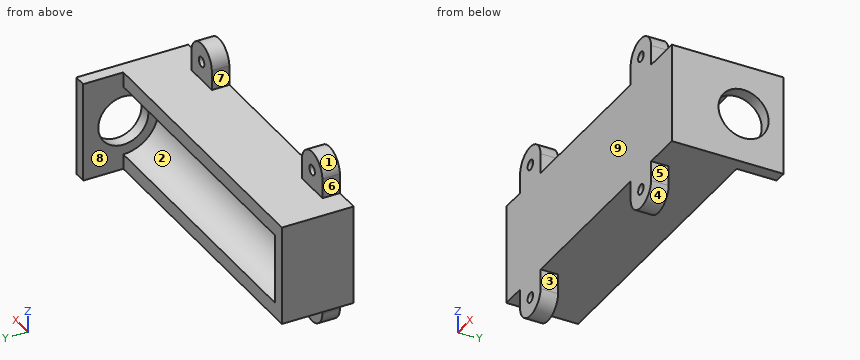
```python
from build123d import *

# Parameters (mm, degrees)
BOSS_EXTRUDE1_DEPTH     = 55.3
SKETCH3_W               = 40
SKETCH3_H               = 19
BOSS_EXTRUDE2_DEPTH     = 5
SKETCH5_R               = 10
CUT_EXTRUDE1_DEPTH      = 10
SKETCH6_W               = 15
SKETCH6_H               = 15
SKETCH6_R               = 2
BOSS_EXTRUDE3_DEPTH     = 5
BOSS_EXTRUDE3_2_DEPTH   = 5
BOSS_EXTRUDE3_3_DEPTH   = 5
BOSS_EXTRUDE3_4_DEPTH   = 5
FILLET5_R               = 7
FILLET2_R               = 7
FILLET3_R               = 7
FILLET4_R               = 7
BOSS_EXTRU_1_START      = 110.6
BOSS_EXTRU_1_DEPTH      = 110.6
ESQUISSE11_W            = 40
ESQUISSE11_H            = 9.66
BOSS_EXTRU_5_DEPTH      = 120.6
ESQUISSE12_R            = 2.003722313
ESQUISSE12_R_2          = 2
BOSS_EXTRU_6_DEPTH      = 7
ESQUISSE13_W            = 97.971196864
ESQUISSE13_H            = 26.942074747
ENL_V_MAT_EXTRU_2_DEPTH = 20
ESQUISSE16_R            = 2
ENL_V_MAT_EXTRU_3_DEPTH = 20
BOSS_EXTRU_7_DEPTH      = 5


with BuildPart() as part:
    # Sketch1 → Boss-Extrude1 (new, symmetric)
    with BuildSketch(Plane(origin=(0, 0, 0), x_dir=(0, 0, -1), z_dir=(1, 0, 0))):
        with BuildLine():
            ThreePointArc((-15, 0), (0, -15), (15, 0))
            Line((15, 0), (20, 0))
            Line((20, 0), (20, -19))
            Line((20, -19), (-20, -19))
            Line((-20, -19), (-20, 0))
            Line((-20, 0), (-15, 0))
        make_face()
    extrude(amount=BOSS_EXTRUDE1_DEPTH, both=True)

    # Sketch3 → Boss-Extrude2 (add)
    with BuildSketch(Plane(origin=(55.3, 0, 0), x_dir=(0, 0, -1), z_dir=(1, 0, 0))):
        with Locations((0, -9.5)):
            Rectangle(SKETCH3_W, SKETCH3_H)
    boss_extrude2 = extrude(amount=BOSS_EXTRUDE2_DEPTH)

    # Mirror1: Boss-Extrude2 across plane
    add(boss_extrude2.mirror(Plane(origin=(0, 0, 0), x_dir=(0, 0, 1), z_dir=(1, 0, 0))))

    # Sketch5 → Cut-Extrude1 (cut)
    with BuildSketch(Plane(origin=(60.3, 0, 0), x_dir=(0, 0, -1), z_dir=(1, 0, 0))):
        Circle(SKETCH5_R)
    extrude(amount=-CUT_EXTRUDE1_DEPTH, mode=Mode.SUBTRACT)

    # Esquisse3 → Boss.-Extru.1 (add)
    with BuildSketch(Plane(origin=(-55.3, 0, 0), x_dir=(0, 0, -1), z_dir=(1, 0, 0)).offset(BOSS_EXTRU_1_START)):
        with BuildLine():
            Line((-15, 0), (-14, 0))
            ThreePointArc((-14, 0), (0, -14), (14, 0))
            Line((14, 0), (15, 0))
            ThreePointArc((15, 0), (0, -15), (-15, 0))
        make_face()
    extrude(amount=-BOSS_EXTRU_1_DEPTH)



with BuildPart() as body_2:
    # Sketch6 → Boss-Extrude3 (new body)
    with BuildSketch(Plane.XZ.offset(19)):
        with Locations((37.8, 27.5)):
            Rectangle(SKETCH6_W, SKETCH6_H)
        with Locations(Location((37.8, 27.5, 0), (0, 0, 270))):
            Circle(SKETCH6_R, mode=Mode.SUBTRACT)
    extrude(amount=-BOSS_EXTRUDE3_DEPTH)

    # Fillet5
    fillet5_edges = [body_2.edges().sort_by_distance(p)[0] for p in [
        (30.3, -16.5, 35),
        (45.3, -16.5, 35),
    ]]
    fillet(fillet5_edges, radius=FILLET5_R)


with BuildPart() as body_3:
    # Sketch6 → Boss-Extrude3 2 (new body)
    with BuildSketch(Plane.XZ.offset(19)):
        with Locations((-42.8, 27.5)):
            Rectangle(SKETCH6_W, SKETCH6_H)
        with Locations(Location((-42.8, 27.5, 0), (0, 0, 270))):
            Circle(SKETCH6_R, mode=Mode.SUBTRACT)
    extrude(amount=-BOSS_EXTRUDE3_2_DEPTH)

    # Fillet2
    fillet2_edges = [body_3.edges().sort_by_distance(p)[0] for p in [
        (-35.3, -16.5, 35),
        (-50.3, -16.5, 35),
    ]]
    fillet(fillet2_edges, radius=FILLET2_R)


with BuildPart() as body_4:
    # Sketch6 → Boss-Extrude3 3 (new body)
    with BuildSketch(Plane.XZ.offset(19)):
        with Locations((37.8, -27.5)):
            Rectangle(SKETCH6_W, SKETCH6_H)
        with Locations(Location((37.8, -27.5, 0), (0, 0, 90))):
            Circle(SKETCH6_R, mode=Mode.SUBTRACT)
    extrude(amount=-BOSS_EXTRUDE3_3_DEPTH)

    # Fillet4
    fillet4_edges = [body_4.edges().sort_by_distance(p)[0] for p in [
        (30.3, -16.5, -35),
        (45.3, -16.5, -35),
    ]]
    fillet(fillet4_edges, radius=FILLET4_R)


with BuildPart() as body_5:
    # Sketch6 → Boss-Extrude3 4 (new body)
    with BuildSketch(Plane.XZ.offset(19)):
        with Locations((-42.8, -27.5)):
            Rectangle(SKETCH6_W, SKETCH6_H)
        with Locations(Location((-42.8, -27.5, 0), (0, 0, 90))):
            Circle(SKETCH6_R, mode=Mode.SUBTRACT)
    extrude(amount=-BOSS_EXTRUDE3_4_DEPTH)

    # Fillet3
    fillet3_edges = [body_5.edges().sort_by_distance(p)[0] for p in [
        (-50.3, -16.5, -35),
        (-35.3, -16.5, -35),
    ]]
    fillet(fillet3_edges, radius=FILLET3_R)


with BuildPart() as part_1:
    add(part.part)

    add(body_2.part)  # Boss.-Extru.5 merges body 2

    add(body_3.part)  # Boss.-Extru.5 merges body 3

    add(body_4.part)  # Boss.-Extru.5 merges body 4

    add(body_5.part)  # Boss.-Extru.5 merges body 5
    # Esquisse11 → Boss.-Extru.5 (add)
    with BuildSketch(Plane.ZY.offset(60.3)):
        with Locations((0, -23.83)):
            Rectangle(ESQUISSE11_W, ESQUISSE11_H)
    extrude(amount=-BOSS_EXTRU_5_DEPTH)

    # Esquisse12 → Boss.-Extru.6 (add)
    # profile 1 of 4: a face of its own
    with BuildSketch(Plane.XZ.offset(28.66)):
        with BuildLine():
            Line((-50.3, 28), (-50.3, 20))
            Line((-50.3, 20), (-35.3, 20))
            Line((-35.3, 20), (-35.3, 28))
            ThreePointArc((-35.3, 28), (-42.8, 35.016648189), (-50.3, 28))
        make_face()
        with Locations(Location((-42.8, 27.5, 0), (0, 0, 270))):
            Circle(ESQUISSE12_R, mode=Mode.SUBTRACT)
    # profile 2 of 4: a face of its own
    with BuildSketch(Plane.XZ.offset(28.66)):
        with BuildLine():
            Line((-35.3, -20), (-50.3, -20))
            Line((-50.3, -20), (-50.3, -28))
            ThreePointArc((-50.3, -28), (-42.8, -35.016648189), (-35.3, -28))
            Line((-35.3, -28), (-35.3, -20))
        make_face()
    # profile 3 of 4: a face of its own
    with BuildSketch(Plane.XZ.offset(28.66)):
        with BuildLine():
            Line((45.3, -20), (30.3, -20))
            Line((30.3, -20), (30.3, -28))
            ThreePointArc((30.3, -28), (37.8, -35.016648189), (45.3, -28))
            Line((45.3, -28), (45.3, -20))
        make_face()
        with Locations(Location((37.8, -27.5, 0), (0, 0, 90))):
            Circle(ESQUISSE12_R_2, mode=Mode.SUBTRACT)
    # profile 4 of 4: a face of its own
    with BuildSketch(Plane.XZ.offset(28.66)):
        with BuildLine():
            Line((30.3, 28), (30.3, 20))
            Line((30.3, 20), (45.3, 20))
            Line((45.3, 20), (45.3, 28))
            ThreePointArc((45.3, 28), (37.8, 35.016648189), (30.3, 28))
        make_face()
        with Locations(Location((37.8, 27.5, 0), (0, 0, 270))):
            Circle(ESQUISSE12_R_2, mode=Mode.SUBTRACT)
    extrude(amount=-BOSS_EXTRU_6_DEPTH)

    # Esquisse13 → Enlèv. mat.-Extru.2 (cut)
    with BuildSketch(Plane(origin=(0, 0, 0), x_dir=(1, 0, 0), z_dir=(0, 1, 0))):
        Polygon((-50.3, -20), (-50.3, -48.328087832), (45.678803054, -48.328087832), (45.3, -20), align=None)
        with Locations((-1.314401568, 33.471037373)):
            Rectangle(ESQUISSE13_W, ESQUISSE13_H)
    extrude(amount=-ENL_V_MAT_EXTRU_2_DEPTH, mode=Mode.SUBTRACT)

    # Esquisse16 → Enlèv. mat.-Extru.3 (cut)
    with BuildSketch(Plane.XZ.offset(28.66)):
        with Locations(Location((-42.8, -27.5, 0), (0, 0, 270))):
            Circle(ESQUISSE16_R)
    extrude(amount=-ENL_V_MAT_EXTRU_3_DEPTH, mode=Mode.SUBTRACT)

    # Esquisse18 → Boss.-Extru.7 (add)
    with BuildSketch(Plane(origin=(60.3, 0, 0), x_dir=(0, 0, -1), z_dir=(1, 0, 0))):
        with BuildLine():
            Line((-20, 0), (-20, 16))
            Line((-20, 16), (20, 16))
            Line((20, 16), (20, 0))
            Line((20, 0), (10, 0))
            ThreePointArc((10, 0), (0, 10), (-10, 0))
            Line((-10, 0), (-20, 0))
        make_face()
    extrude(amount=-BOSS_EXTRU_7_DEPTH)


solid = part_1.part
```
CAD build for the part. Positions are in the model's coordinates, mm. Face numbers are marked on the shaded views. A direction names the side the tool comes from. Round coordinates to 2 decimals unless told otherwise and drop trailing zeros. Loops run counter-clockwise (first coordinate to the right, second up) from the corner with the lowest first, then second, coordinate; pieces in that order, holes last. Notation, with made-up numbers: (58.5, -15.75) - (111.5, -15.75) arc R16 ccw to (111.5, -4.75) - close; hole circle Ø5 at (53.5, 56). An arc over 180 degrees is marked (long way). Return JSON: item names as keys, results as strings. Group by question number.
Q1. Two-plate mould, pull along Z, no slides. Class the marked faces 1, 2, 3 and 4: +Z half, -Z half, draft (parallel to the pull), parting line (faces both ways), or undercut.
Q2. Flat gauge pins, fed straight in: pin 1 Ø22.5 at (x, y) = (15, -8) entering from +Z; pin 2 Ø2 at (y, z) = (-24.5, 24) entering from +X; pin 3 Ø12 at (y, z) = (0, 0) entering from +X. Where does each tip first touch, or does it go through?
Q3. Tool access for the marked faces 5, 6, 7, 8 and 9: list every direction of +Z, -Z, +X, -X, +Y, -Y with a clear straight run to the whole face (end or side of a thin tool).
Q4. Band-saw the part on A-A on z = 22. Give the cut face in (x, y), plus the area to 3 significant figures.
Q5. Band-saw the part on D-D on z = -17. Give the cut face in (x, y), plus the area to 3 significant figures.
Q6. Band-saw the part on C-C on y = 3. Give the cut face in (x, z), plus the area to 3 significant figures.
Q7. Band-saw the part on B-B on x = 37.8. Give the cut face in (y, z), plus the area to 3 significant figures.
Q8. Drill centre lines: line 1 along X through (y, z) = (-27, 27.5); line 2 along Y through (x, z) = (59, 0); line 3 along Z through (x, y) = (37, -26). Where is each one in solid material? Low to high. Write a range as [from, to].
Solutions:
{
 "1": {"face 1": "+Z half", "face 2": "undercut", "face 3": "draft", "face 4": "-Z half"},
 "2": {"pin 1": "stops at z = 20", "pin 2": "stops at x = 45.3", "pin 3": "stops at x = -55.3"},
 "3": {"face 5": "-Z, +X, +Y, -Y", "face 6": "+Z, -X, +Y, -Y", "face 7": "+Z, +Y, -Y", "face 8": "+Y", "face 9": "+Z, -Z, +X, -X, -Y"},
 "4": {"outline": "(-50.3, -28.66) - (-35.3, -28.66) - (-35.3, -21.66) - (-50.3, -21.66) - close; (30.3, -28.66) - (45.3, -28.66) - (45.3, -21.66) - (30.3, -21.66) - close", "area": "210 mm^2"},
 "5": {"outline": "(-60.3, -28.66) - (60.3, -28.66) - (60.3, 16) - (55.3, 16) - (55.3, 0) - (-60.3, 0) - close", "area": "3,540 mm^2"},
 "6": {"outline": "(55.3, -20) - (60.3, -20) - (60.3, -9.54) - (55.3, -9.54) - close; (55.3, 9.54) - (60.3, 9.54) - (60.3, 20) - (55.3, 20) - close", "area": "105 mm^2"},
 "7": {"outline": "(-28.66, -35.02) - (-21.66, -35.02) - (-21.66, -29.5) - (-28.66, -29.5) - close; (-28.66, -25.5) - (-21.66, -25.5) - (-21.66, -20) - (0, -20) - (0, -14) arc R14 cw to (0, 14) - (0, 20) - (-21.66, 20) - (-21.66, 25.5) - (-28.66, 25.5) - close; (-28.66, 29.5) - (-21.66, 29.5) - (-21.66, 35.02) - (-28.66, 35.02) - close", "area": "993 mm^2"},
 "8": {"line 1": "x = [-50.3, -44.8], [-40.8, -35.3], [30.3, 35.8], [39.8, 45.3]", "line 2": "y = [-28.66, -10], [10, 16]", "line 3": "z = [-34.97, -29.33], [-25.67, 25.67], [29.33, 34.97]"}
}
